from build123d import *

# Parameters (mm, degrees)
BOSS_EXTRUDE1_DEPTH = 15
SKETCH2_W           = 12
SKETCH2_H           = 10
BOSS_EXTRUDE2_DEPTH = 12.6
FILLET1_R           = 1
BOSS_EXTRUDE3_DEPTH = 8.7
SKETCH4_R           = 2.5
BOSS_EXTRUDE4_DEPTH = 1.3
SKETCH5_R           = 0.5
BOSS_EXTRUDE5_DEPTH = 4.2


with BuildPart() as part:
    # Sketch1 → Boss-Extrude1 (new body)
    with BuildSketch(Plane.XY):
        with BuildLine():
            Line((-3.45, 5), (3.45, 5))
            ThreePointArc((3.45, 5), (6, 0), (3.45, -5))
            Line((3.45, -5), (-3.45, -5))
            ThreePointArc((-3.45, -5), (-6, 0), (-3.45, 5))
        make_face()
    extrude(amount=BOSS_EXTRUDE1_DEPTH)

    # Sketch2 → Boss-Extrude2 (add)
    with BuildSketch(Plane.XY.offset(15)):
        Rectangle(SKETCH2_W, SKETCH2_H)
    extrude(amount=BOSS_EXTRUDE2_DEPTH)

    # Fillet1
    fillet1_edges = [part.edges().sort_by_distance(p)[0] for p in [
        (6, -5, 21.3),
        (6, 5, 21.3),
        (-6, 5, 21.3),
        (-6, -5, 21.3),
    ]]
    fillet(fillet1_edges, radius=FILLET1_R)

    # Sketch3 → Boss-Extrude3 (add)
    with BuildSketch(Plane.XY.offset(27.6)):
        with BuildLine():
            Line((1, 1.118033989), (1, -1.118033989))
            ThreePointArc((1, -1.118033989), (-1.5, 0), (1, 1.118033989))
        make_face()
    extrude(amount=BOSS_EXTRUDE3_DEPTH)

    # Sketch4 → Boss-Extrude4 (add)
    with BuildSketch(Plane(origin=(0, 0, 0), x_dir=(-1, 0, 0), z_dir=(0, 0, -1))):
        Circle(SKETCH4_R)
    extrude(amount=BOSS_EXTRUDE4_DEPTH)

    # Sketch5 → Boss-Extrude5 (add)
    with BuildSketch(Plane(origin=(0, 0, -1.3), x_dir=(-1, 0, 0), z_dir=(0, 0, -1))):
        Circle(SKETCH5_R)
    extrude(amount=BOSS_EXTRUDE5_DEPTH)


solid = part.part
Check sheet for the modelled part. Datum: model origin and axes. Units: mm. A direction names the side the tool comes from. Give positions to 0.01 mm unless a question says otherwise; leave off trailing zeros. Loops run counter-clockwise (first coordinate to the right, second up) from the corner with the lowest first, then second, coordinate; pieces in that order, holes last. Notation, with made-up numbers: M 70,-22 L 89,-22 A27 ccw 89,-4 Z; hole C 79,53.25 d10. An arc over 180 degrees is marked long. Return JSON: item names as keys, results as strings. Group by question number.
1. Cross-section at A-A on x = 0. Record the boundary of the cut face in (y, z), plus the area to 3 significant figures.
2. Go/stop test with flat-tipped pins: pin 1 (2 mm diameter, centred on x = 4.5, y = 2.5, fed in from -Z); pin 2 (1.1 mm diameter, centred on y = -0.5, z = 31, fed in from +X). Record where each tip stops, or that it passes through.
3. Tool access check on faces 1 (the flat face through (-5, 4, 15)), 2 (the cylindrical face through (-6, 0, 7)), 3 (the flat face through (5, -4, 15)), 4 (the flat face through (-5, -4, 15)). Record the directions out of +Z, -Z, +X, -X, +Y, -Y that give a thin tool (end or side, any length) a straight path to the whole face; none if there is none.
4. Thickness scan on L1, parallel to Z at x = -2.25, y = -1.5; L2, parallel to Z at x = 1.25, y = 0.75; L3, parallel to X at y = 3.25, z = 11. Record the ranges inside material, lowest first.
5. Cross-section at B-B on z = 28.5. Record the boundary of the cut face in (x, y), plus the area to 3 significant figures.
6. Cross-section at C-C on y = 2. Record the boundary of the cut face in (x, z).
7. Cross-section at D-D on z = 1. Record the boundary of the cut face in (x, y), plus the area to 3 significant figures.
Return value:
{
 "1": {"outline": "M -5,0 L -2.5,0 L -2.5,-1.3 L -0.5,-1.3 L -0.5,-5.5 L 0.5,-5.5 L 0.5,-1.3 L 2.5,-1.3 L 2.5,0 L 5,0 L 5,27.6 L 1.5,27.6 L 1.5,36.3 L -1.5,36.3 L -1.5,27.6 L -5,27.6 Z", "area": "313 mm^2"},
 "2": {"pin 1": "z = 0", "pin 2": "x = 1"},
 "3": {"face 1": "-Z, -X, +Y", "face 2": "-Z, -X", "face 3": "-Z, +X, -Y", "face 4": "-Z, -X, -Y"},
 "4": {"L1": "0 to 27.6", "L2": "-1.3 to 27.6", "L3": "-5.08 to 5.08"},
 "5": {"outline": "M 1,-1.12 L 1,1.12 A1.5 ccw long Z", "area": "6.29 mm^2"},
 "6": {"outline": "M -6,15 L -5.67,15 L -5.67,0 L -1.5,0 L -1.5,-1.3 L 1.5,-1.3 L 1.5,0 L 5.67,0 L 5.67,15 L 6,15 L 6,27.6 L -6,27.6 Z"},
 "7": {"outline": "M -3.45,-5 L 3.45,-5 A6.18 ccw 3.45,5 L -3.45,5 A6.18 ccw Z", "area": "105 mm^2"}
}
